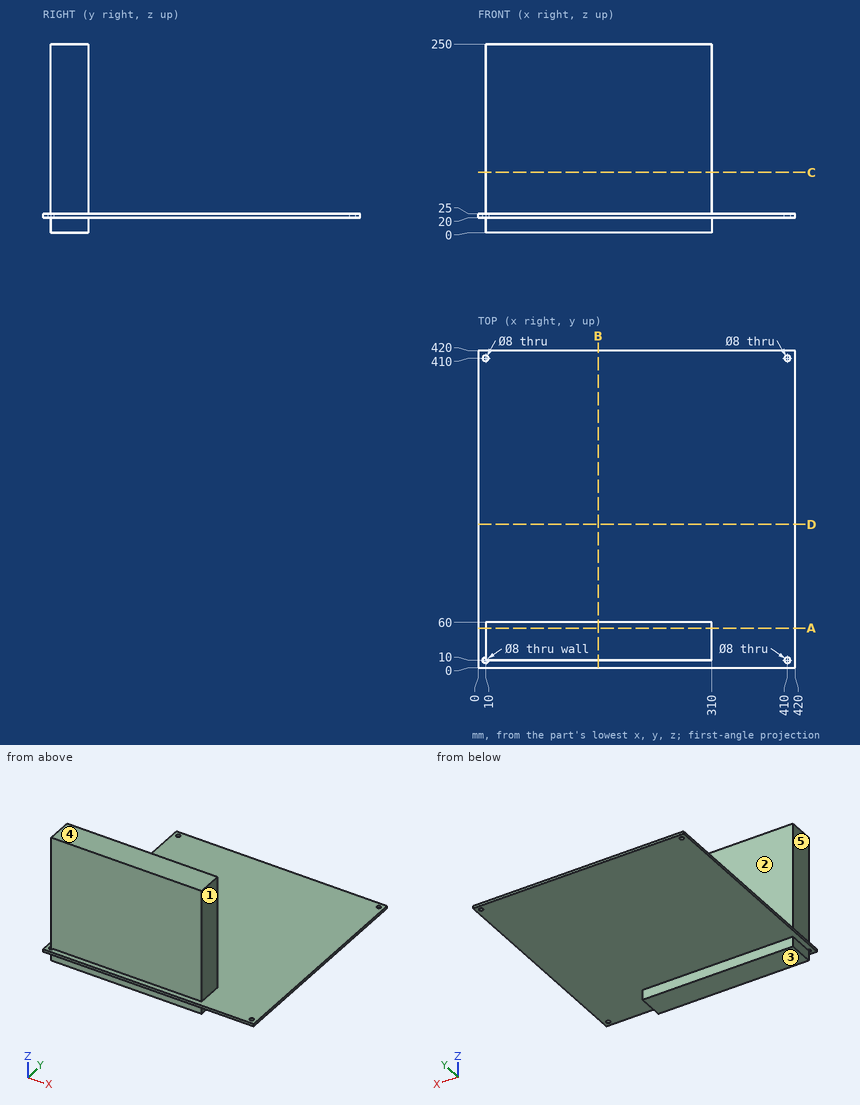
Study the drawing (mm; zero at the part's minimum x, y, z) and answer. A direction names the side the tool comes from. Round coordinates to 2 decimals unless told otherwise and drop trailing zeros. Loops run counter-clockwise (first coordinate to the right, second up) from the corner with the lowest first, then second, coordinate; pieces in that order, holes last.
Q1. Section C-C, the plane z = 80 is taken. Determine the outline of the cut face in (x, y), then the cut area to 3 significant figures.
Q2. Section A-A, the plane y = 52.5 is taken. Determine the outline of the cut face in (x, z).
Q3. Find the intervals of material crossed by line 1 (Y direction, x = 410, z = 23.55); line 2 (Z direction, x = 54.5, y = 117.5), in increasing order.
Q4. Section B-B, the plane x = 159 is taken. Determine the outline of the cut face in (y, z), then the cut area to 4 significant figures.
Q5. Which of the six approach directions +Z, -Z, +X, -X, +Y, -Y give full straight-line access (tool end or side, diameter ignored) to the marked faces 1 and 2?
Q6. Given pin 1 Ø5 at (x, z) = (291, 160.5) entering from +Y; pin 2 Ø4 at (y, z) = (45, 155) entering from -X; pin 3 Ø3 at (x, y) = (268, 158.5) entering from +Z, each flat-ended and moving along its own axis, determine where each tip first touches the part or whether it passes through.
Q7. For a pull along Z with two mould halves and no side action, classify the marked faces 3, 4 and 5 as released by +Z, released by -Z, zero draft, split by the parting line, or undercut.
Q8. Section D-D, the plane y = 190 is taken. Determine the outline of the cut face in (x, z), then the cut area to 3 significant figures.
Completed:
1. outline: (10, 10) - (310, 10) - (310, 60) - (10, 60) - close
1. area: 15,000 mm2
2. outline: (0, 20) - (10, 20) - (10, 0) - (310, 0) - (310, 20) - (420, 20) - (420, 25) - (310, 25) - (310, 250) - (10, 250) - (10, 25) - (0, 25) - close
3. line 1: y = 0 to 6, 14 to 406, 414 to 420
3. line 2: z = 20 to 25
4. outline: (0, 20) - (10, 20) - (10, 0) - (60, 0) - (60, 20) - (420, 20) - (420, 25) - (60, 25) - (60, 250) - (10, 250) - (10, 25) - (0, 25) - close
4. area: 14,350 mm2
5. face 1: +Z, +X, +Y, -Y
5. face 2: +Z, +X, -X, +Y
6. pin 1: stops at y = 60
6. pin 2: stops at x = 10
6. pin 3: stops at z = 25
7. face 3: released by -Z
7. face 4: released by +Z
7. face 5: zero draft
8. outline: (0, 20) - (420, 20) - (420, 25) - (0, 25) - close
8. area: 2,100 mm2
